from build123d import *

# Parameters (mm, degrees)
F2_SIZE = 20


with BuildPart() as f1:
    # F0 (on Front) → F1 (revolve)
    with BuildSketch(Plane.XZ):
        with BuildLine():
            Line((100, 162.432451), (100, 482.432451))
            Line((100, 482.432451), (0, 482.432451))
            Line((0, 482.432451), (0, -217.567549))
            Line((0, -217.567549), (400, -67.567549))
            Line((400, -67.567549), (400, 82.432451))
            Line((400, 82.432451), (180, 82.432451))
            ThreePointArc((180, 82.432451), (123.431458, 105.863908), (100, 162.432451))
        make_face()
    revolve(axis=Axis((0, 0, 132.432451), (0, 0, -1)))

    # F2
    f2_edges = [f1.edges().sort_by_distance(p)[0] for p in [
        (-100, 0, 482.432451),
    ]]
    chamfer(f2_edges, length=F2_SIZE)


solid = f1.part
Verification items for the finished model (mm, model axes). A direction names the side the tool comes from. Coordinates: 2 decimals unless noted, no trailing zeros. Order: outer loops, then holes, each group sorted by start corner. A loop starts at its lowest first (then second) coordinate and runs counter-clockwise, first axis right, second up. Notation, with made-up numbers: (58, 57) -> (92, 57) arc R26 ccw to (92, 92) -> close; hole circle Ø6 at (0.5, 19.25). An arc over 180 degrees is marked (long way). Put each result on its own line as item: value. Start each with the question number.
1. Material ranges on L1, parallel to Y at x = 4, z = 319.5; L2, parallel to Z at x = -307.5, y = 255; L3, parallel to X at y = -50, z = 32, recorded low to high. Write a range as [from, to].
2. Go/stop test with flat-tipped pins: pin 1 Ø4 at (x, y) = (87.5, -29) entering from +Z; pin 2 Ø8 at (x, z) = (-264, 32.5) entering from +Y; pin 3 Ø12 at (x, z) = (-165.5, 36.5) entering from -Y. Record where each tip stops, or that it passes through.
3. Cross-section at B-B, the plane z = -131. Record the boundary of the cut face in (x, y), then the cut area to 3 significant figures.
4. Cross-section at A-A, the plane z = 380. Record the boundary of the cut face in (x, y), then the cut area to 3 significant figures.
5. Access from +Z, -Z, +X, -X, +Y, -Y to the whole of each face (thin tool, end or side, straight path). Record for faces 1 (the cylindrical face through (95.38, -30.04, 314.53)), 2 (the cylindrical face through (381.53, -120.15, 8.48)).
Computed:
1. L1: [-99.92, 99.92]
1. L2: [-67.76, 82.43]
1. L3: [-396.86, 396.86]
2. pin 1: z = 472.25
2. pin 2: y = 303.97
2. pin 3: y = -366.82
3. outline: circle Ø461.69 at (0, 0)
3. area: 167,000 mm2
4. outline: circle Ø200 at (0, 0)
4. area: 31,400 mm2
5. face 1: +Z
5. face 2: +Z, -Z
